Part model, mm, in its own coordinate system. A direction names the side the tool comes from. Coordinates: 2 decimals unless noted, no trailing zeros. Loops run counter-clockwise (first coordinate to the right, second up) from the corner with the lowest first, then second, coordinate; pieces in that order, holes last. Notation, with made-up numbers: (6.5, 47) -> (19.5, 47) arc R32 ccw to (19.5, 77) -> close; hole circle Ø1 at (62.25, 53). An arc over 180 degrees is marked (long way). One line per item, written item: value. Start each with the question number.
from build123d import *

# Parameters (mm, degrees)
CHAMFER1_SIZE      = 0.35
CUT_EXTRUDE1_START = -1.8000001
CUT_EXTRUDE1_DEPTH = 2.8000001
FILLET1_R          = 0.2


with BuildPart() as part:
    # Sketch1 → Revolve1 (revolve)
    with BuildSketch(Plane(origin=(0, 0, 0), x_dir=(0, 0, -1), z_dir=(1, 0, 0)), mode=Mode.PRIVATE) as revolve1_sk:
        with BuildLine():
            Line((16, 0), (16, 2))
            Line((16, 2), (0, 2))
            Line((0, 2), (0, 3.75))
            Line((0, 3.75), (-0.4, 3.75))
            ThreePointArc((-0.4, 3.75), (-1.845304899, 3.217657748), (-2.6, 1.875))
            Line((-2.6, 1.875), (-2.6, 0))
            Line((-2.6, 0), (16, 0))
        make_face()
    revolve(revolve1_sk.sketch.rotate(Axis((0, 0, 30.809969789), (0, 0, -1)), 90), axis=Axis((0, 0, 30.809969789), (0, 0, -1)))

    # Chamfer1
    chamfer1_edges = [part.edges().sort_by_distance(p)[0] for p in [
        (-2, 0, -16),
    ]]
    chamfer(chamfer1_edges, length=CHAMFER1_SIZE)

    # Sketch2 → Cut-Revolve1 (revolve, cut)
    with BuildSketch(Plane(origin=(0, 0, 0), x_dir=(0, 0, -1), z_dir=(1, 0, 0)), mode=Mode.PRIVATE) as cut_revolve1_sk:
        Polygon((-2.6, 0), (-2.6, 1.25), (-0.8, 1.25), (-0.078312164, 0), align=None)
    revolve(cut_revolve1_sk.sketch.rotate(Axis((0, 0, 2.452500839), (0, 0, -1)), 90), axis=Axis((0, 0, 2.452500839), (0, 0, -1)), mode=Mode.SUBTRACT)

    # Cut-Extrude1: read off the stored shape, not the designer's step
    # Cut-Extrude1 outline → Cut-Extrude1 (cut)
    with BuildSketch(Plane.XY.offset(2.6).offset(CUT_EXTRUDE1_START)):
        with BuildLine():
            Line((1.25, 0), (1.25, 0.721687836))
            Line((1.25, 0.721687836), (0.625, 1.082531755))
            ThreePointArc((0.625, 1.082531755), (1.082531755, 0.625), (1.25, 0))
        make_face()
        with BuildLine():
            ThreePointArc((-0.625, 1.082531755), (0, 1.25), (0.625, 1.082531755))
            Line((0.625, 1.082531755), (0, 1.443375673))
            Line((0, 1.443375673), (-0.625, 1.082531755))
        make_face()
        with BuildLine():
            Line((1.25, -0.721687836), (1.25, 0))
            ThreePointArc((1.25, 0), (1.082531755, -0.625), (0.625, -1.082531755))
            Line((0.625, -1.082531755), (1.25, -0.721687836))
        make_face()
        with BuildLine():
            ThreePointArc((-1.25, 0), (-1.082531755, 0.625), (-0.625, 1.082531755))
            Line((-0.625, 1.082531755), (-1.25, 0.721687836))
            Line((-1.25, 0.721687836), (-1.25, 0))
        make_face()
        with BuildLine():
            Line((0, -1.443375673), (0.625, -1.082531755))
            ThreePointArc((0.625, -1.082531755), (0, -1.25), (-0.625, -1.082531755))
            Line((-0.625, -1.082531755), (0, -1.443375673))
        make_face()
        with BuildLine():
            ThreePointArc((-0.625, -1.082531755), (-1.082531755, -0.625), (-1.25, 0))
            Line((-1.25, 0), (-1.25, -0.721687836))
            Line((-1.25, -0.721687836), (-0.625, -1.082531755))
        make_face()
    extrude(amount=CUT_EXTRUDE1_DEPTH, mode=Mode.SUBTRACT)

    # Cut-Extrude1 2 outline → Cut-Extrude1 2 (revolve)
    with BuildSketch(Plane.XZ):
        Polygon((1.443375738, 0.911645534), (1.249999957, 0.799999975), (1.443375673, 0.7999999), align=None)
    revolve(axis=Axis((0, 0, 0), (0, 0, 1)))

    # Fillet1
    fillet1_edges = [part.edges().sort_by_distance(p)[0] for p in [
        (-2, 0, 0),
    ]]
    fillet(fillet1_edges, radius=FILLET1_R)


solid = part.part
1) Tool access for faces 1 (the flat face through (-2, 2, 0)), 2 (the flat face through (-1.25, 0, 2)), 3 (the cylindrical face through (2.02, -3.16, 0.2)): list every direction of +Z, -Z, +X, -X, +Y, -Y with a clear straight run to the whole face (end or side of a thin tool).
2) Slice it at A-A (z = -10). Give the cut face in (x, y), then the cut area to 3 significant figures.
3) Pin check, flat tips, straight feed: pin 1 Ø1.5 at (x, z) = (1.5, -7) entering from -Y; pin 2 Ø1.2 at (y, z) = (0, 2) entering from +X; pin 3 Ø1.5 at (x, z) = (1.5, -13.5) entering from +Y. Stop position of each tip, or through.
4) Probe line 1 (Y direction, x = -0.25, z = 1.75); line 2 (X direction, y = 0.25, z = 1.25); line 3 (Y direction, x = 0, z = -13.25). List the from-to ranges inside material, lowest first. Write a range as from..to.
5) Pull direction X, two halves, no side cores. Call faces 4 (the flat face through (1.25, 0, 2)), 5 (the cylindrical face through (0, 2, -8)), 6 (the flat face through (0, 0, -16)): +X half, -X half, draft (parallel to the pull), parting line (faces both ways), or undercut.
Check sheet entries:
1. face 1: -Z
1. face 2: +Z
1. face 3: +Z, -Z
2. outline: circle Ø4 at (0, 0)
2. area: 12.6 mm^2
3. pin 1: stops at y = -1.85
3. pin 2: stops at x = 3.51
3. pin 3: stops at y = 1.85
4. line 1: y = -3.28..-1.3, 1.3..3.28
4. line 2: x = -3.57..-1.25, 1.25..3.57
4. line 3: y = -2..2
5. face 4: undercut
5. face 5: parting line
5. face 6: draft
